from build123d import *

# Parameters (mm, degrees)
F1_DEPTH = 5.08
F2_R     = 5.08
F3_DEPTH = 25.4
F4_R     = 12.7
F5_SIZE  = 2.53999
F6_R     = 2.53999


# Not quite as in the source:
# - a fillet or chamfer is up to 0.001 mm smaller than in the source, because OpenCascade refuses the exact size


with BuildPart() as f1:
    # F0 (on Front) → F1 (new body)
    with BuildSketch(Plane.XZ):
        with BuildLine():
            Line((-12.7, 0), (0, 0))
            Line((0, 0), (0, 12.7))
            ThreePointArc((0, 12.7), (-11.1850810666, 8.4922018267), (-23.0563643922, 9.8648766371))
            Line((-23.0563643922, 9.8648766371), (-38.1, 0))
            Line((-38.1, 0), (-12.7, 0))
        make_face()
        with BuildLine():
            Line((0, 12.7), (0, 0))
            Line((0, 0), (12.7, 0))
            ThreePointArc((12.7, 0), (8.4922018267, 11.1850810666), (9.8648766371, 23.0563643922))
            Line((9.8648766371, 23.0563643922), (0, 38.1))
            Line((0, 38.1), (0, 12.7))
        make_face()
        with BuildLine():
            Line((0, -12.7), (0, 0))
            Line((0, 0), (-12.7, 0))
            ThreePointArc((-12.7, 0), (-8.4922018267, -11.1850810666), (-9.8648766371, -23.0563643922))
            Line((-9.8648766371, -23.0563643922), (0, -38.1))
            Line((0, -38.1), (0, -12.7))
        make_face()
        with BuildLine():
            Line((12.7, 0), (0, 0))
            Line((0, 0), (0, -12.7))
            ThreePointArc((0, -12.7), (11.1850810666, -8.4922018267), (23.0563643922, -9.8648766371))
            Line((23.0563643922, -9.8648766371), (38.1, 0))
            Line((38.1, 0), (12.7, 0))
        make_face()
    extrude(amount=F1_DEPTH)

    # F2 (on face) → F3 (cut)
    with BuildSketch(Plane.XZ.offset(5.08)):
        Circle(F2_R)
    extrude(amount=-F3_DEPTH, mode=Mode.SUBTRACT)

    # F4
    f4_edges = [f1.edges().sort_by_distance(p)[0] for p in [
        (0, -2.54, 12.7),
        (12.7, -2.54, 0),
        (0, -2.54, -12.7),
        (-12.7, -2.54, 0),
    ]]
    fillet(f4_edges, radius=F4_R)

    # F5 (size 2.54 in the source; OpenCascade refuses exactly that, so slightly less here)
    f5_edges = [f1.edges().sort_by_distance(p)[0] for p in [
        (30.578182, 0, -4.932438),
        (30.578182, -5.08, -4.932438),
        (4.932438, 0, 30.578182),
        (4.932438, -5.08, 30.578182),
        (-4.932438, 0, -30.578182),
        (-4.932438, -5.08, -30.578182),
        (-30.578182, 0, 4.932438),
        (-30.578182, -5.08, 4.932438),
    ]]
    chamfer(f5_edges, length=F5_SIZE)

    # F6 (radius 2.54 in the source; OpenCascade refuses exactly that, so slightly less here)
    f6_edges = [f1.edges().sort_by_distance(p)[0] for p in [
        (-5.08, 0, 0),
        (-5.08, -5.08, 0),
    ]]
    fillet(f6_edges, radius=F6_R)


solid = f1.part
Model file for the job. Use its own axes, mm. A direction names the side the tool comes from. Coordinates: 2 decimals unless noted, no trailing zeros. Order: outer loops, then holes, each group sorted by start corner. A loop starts at its lowest first (then second) coordinate and runs counter-clockwise, first axis right, second up. Notation, with made-up numbers: (36.5, -1.75) -> (43.5, -1.75) arc R14 ccw to (43.5, 9.25) -> close; hole circle Ø1 at (47.5, 54.5). An arc over 180 degrees is marked (long way). Return JSON: item names as keys, results as strings. Group by question number.
Item 1: Tool access for faces 4 (the flat face through (0, -3, 28)), 5 (the cylindrical face through (-3.261, -2.576, 12.604)), 6 (the flat face through (0, -3, -28)), 7 (the flat face through (-28, -3, 0)), 8 (the cylindrical face through (3.09, -2.58, -12.8)): list every direction of +Z, -Z, +X, -X, +Y, -Y with a clear straight run to the whole face (end or side of a thin tool).
Item 2: Wall check: line 1 along Z through (x, y) = (-24, -4.75); line 2 along Z through (x, y) = (27, -4.8); line 3 along X through (y, z) = (-0.35, 3). Give the ranges that are in metal, low to high. Write a range as [from, to].
Item 3: Saw through at D-D on z = -13.5. Write the cut outline in (x, y).
Item 4: Saw through at A-A on y = -0.95. Write the cut outline in (x, z), then the cut area to 3 significant figures.
Item 5: Saw through at C-C on z = -22. Write the cut outline in (x, y), then the cut area to 3 significant figures.
Item 6: Flat gauge pins, fed straight in: P1, Ø4, axis at x = 29, z = -6.5, coming from the +Y side; P2, Ø1.5, axis at x = -30, y = -1.5, coming from the -Z side; P3, Ø1.5, axis at y = -3, z = 28, coming from the -X side. Where does each tip first touch, or does it go through?
Item 7: Pull direction Z, two halves, no side cores. Call faces 1 (the cylindrical face through (8.344, -2.504, 15.74)), 2 (the cylindrical face through (15.74, -2.504, -8.344)), 3 (the flat face through (4.553, -1.288, 28.873)): pulls with the +Z half, pulls with the -Z half, needs draft (parallel to the pull), parting line crosses it, or undercut.
Values found:
{
 "1": {"face 4": "+Z, -X, +Y, -Y", "face 5": "+Z, +Y, -Y", "face 6": "-Z, +X, +Y, -Y", "face 7": "-Z, -X, +Y, -Y", "face 8": "-Z, +Y, -Y"},
 "2": {"line 1": "z = [0, 6.6]", "line 2": "z = [-4.58, 0]", "line 3": "x = [-29.53, -5.58], [5.58, 12.9]"},
 "3": {"outline": "(-8.31, -5.08) -> (2.53, -5.08) -> (2.53, 0) -> (-8.31, 0) -> close"},
 "4": {"outline": "(-35.2, 0) -> (-21.1, 0) arc R12.7 cw to (-8.5, -11.11) arc R25.4 cw to (-9.24, -21.11) -> (0, -35.2) -> (0, -21.1) arc R12.7 cw to (11.11, -8.5) arc R25.4 cw to (21.11, -9.24) -> (35.2, 0) -> (21.1, 0) arc R12.7 cw to (8.5, 11.11) arc R25.4 cw to (9.24, 21.11) -> (0, 35.2) -> (0, 21.1) arc R12.7 cw to (-11.11, 8.5) arc R25.4 cw to (-21.11, 9.24) -> close; hole circle Ø11.28 at (0, 0)", "area": "1,010 mm2"},
 "5": {"outline": "(-9.5, -3.42) -> (-7.52, -5.08) -> (0, -5.08) -> (0, 0) -> (-7.52, 0) -> (-9.5, -1.66) -> close", "area": "45.0 mm2"},
 "6": {"P1": "stops at y = -0.99", "P2": "stops at z = 0", "P3": "stops at x = 0"},
 "7": {"face 1": "undercut", "face 2": "pulls with the -Z half", "face 3": "pulls with the +Z half"}
}
